Here's how the part is built. I have some questions about the finished solid (model axes, mm). A direction names the side the tool comes from. Round coordinates to 2 decimals unless told otherwise and drop trailing zeros. Write each loop counter-clockwise with the first axis right and the second up, starting at its lowest first coordinate (ties: lowest second). Pieces come first, ordered by that corner, then holes. Notation, with made-up numbers: (-31.75, -22) - (9.25, -22) arc R24 ccw to (9.25, 12) - close; hole circle Ø5 at (-10, -40). An arc over 180 degrees is marked (long way). Write item = value, one per line. Start each with the question number.
Item 1: Thinking about a two-plate mould opening in X: for faces 4 (the face through (10.57, 51.4, 1.52)), 5 (the face through (46, 39, 1)), 6 (the face through (28, 41.6, 1)), which applies, pulls with the +X half, pulls with the -X half, needs draft (parallel to the pull), parting line crosses it, or undercut?
Item 2: If we section it at D-D (x = 19): Please give me the cut outline in (y, z), and give its area (3 significant figures).
Item 3: If we section it at B-B (z = 10): Please give me the cut outline in (x, y).
Item 4: If we section it at A-A (y = 36.5): Please give me the cut outline in (x, z).
Item 5: Which directions (+Z, -Z, +X, -X, +Y, -Y) give clear straight access to the entire face, cutting with the end or side of a thin tool? Please do faces 1 (the face through (28, 31.6, 1)), 2 (the face through (54, 26, 6)), 3 (the face through (2, 26, 6)).
Item 6: If I drill on line 1 along Y through (x, z) = (2.1, 5); line 2 along X through (y, z) = (6.5, 7); line 3 along Z through (x, y) = (29, 45.5), over which ranges is the centre line in solid material (lowest first)? Write a range as [from, to].
Item 7: If we section it at C-C (z = 4.25): Please give me the cut outline in (x, y).
Item 8: For P1, Ø2, axis at y = 4, z = 5, coming from the +X side; P2, Ø6.5, axis at x = 5, z = 12, coming from the +Y side; P3, Ø0.9, axis at y = 35, z = 1, coming from the -X side; P4, Ø25, axis at x = 22.5, y = 14, coming from the +Z side, each with a flat end and sliding along its axis, tell me the tip position at first contact or that it passes through.
```python
from build123d import *

# Parameters (mm, degrees)
SKETCH_1_W          = 3
SKETCH_1_H          = 26
EXTRUDE_4_DEPTH     = 3
SKETCH_2_W          = 3
SKETCH_2_H          = 26
EXTRUDE_5_DEPTH     = 15
CUT_EXTRUDE_2_DEPTH = 56
FILLET_2_R          = 2


with BuildPart() as part:
    # 草图1 → 凸台-拉伸4 (new body)
    with BuildSketch(Plane.XY):
        with BuildLine():
            Line((10, 26), (3, 26))
            Line((3, 26), (3, 0))
            Line((3, 0), (28, 0))
            Line((28, 0), (28, 4.6))
            ThreePointArc((28, 4.6), (24.535898385, 5.110874707), (21.366750419, 6.6))
            Line((21.366750419, 6.6), (19.65, 6.6))
            ThreePointArc((19.65, 6.6), (16.833273811, 5.433273811), (18, 8.25))
            Line((18, 8.25), (18, 9.966750419))
            ThreePointArc((18, 9.966750419), (16, 16.6), (18, 23.233249581))
            Line((18, 23.233249581), (18, 24.95))
            ThreePointArc((18, 24.95), (16.35, 26.6), (18, 28.25))
            Line((18, 28.25), (18, 31.6))
            Line((18, 31.6), (18, 41.6))
            Line((18, 41.6), (18, 44.95))
            ThreePointArc((18, 44.95), (16.833273811, 47.766726189), (19.65, 46.6))
            Line((19.65, 46.6), (28, 46.6))
            Line((28, 46.6), (28, 52))
            Line((28, 52), (10, 52))
            Line((10, 52), (10, 26))
        make_face()
        with BuildLine():
            Line((28, 4.6), (28, 0))
            Line((28, 0), (53, 0))
            Line((53, 0), (53, 26))
            Line((53, 26), (46, 26))
            Line((46, 26), (46, 52))
            Line((46, 52), (28, 52))
            Line((28, 52), (28, 46.6))
            Line((28, 46.6), (36.35, 46.6))
            ThreePointArc((36.35, 46.6), (38, 48.25), (39.65, 46.6))
            ThreePointArc((39.65, 46.6), (39.166726189, 45.433273811), (38, 44.95))
            Line((38, 44.95), (38, 41.6))
            Line((38, 41.6), (38, 31.6))
            Line((38, 31.6), (38, 28.25))
            ThreePointArc((38, 28.25), (39.166726189, 27.766726189), (39.65, 26.6))
            ThreePointArc((39.65, 26.6), (39.166726189, 25.433273811), (38, 24.95))
            Line((38, 24.95), (38, 23.233249581))
            ThreePointArc((38, 23.233249581), (39.489125293, 20.064101615), (40, 16.6))
            ThreePointArc((40, 16.6), (39.489125293, 13.135898385), (38, 9.966750419))
            Line((38, 9.966750419), (38, 8.25))
            ThreePointArc((38, 8.25), (39.166726189, 7.766726189), (39.65, 6.6))
            ThreePointArc((39.65, 6.6), (38, 4.95), (36.35, 6.6))
            Line((36.35, 6.6), (34.633249581, 6.6))
            ThreePointArc((34.633249581, 6.6), (31.464101615, 5.110874707), (28, 4.6))
        make_face()
        with Locations((54.5, 13)):
            Rectangle(SKETCH_1_W, SKETCH_1_H)
        with Locations((1.5, 13)):
            Rectangle(SKETCH_1_W, SKETCH_1_H)
        with BuildLine():
            ThreePointArc((18, 23.233249581), (22.325451338, 27.173528147), (28, 28.6))
            Line((28, 28.6), (28, 31.6))
            Line((28, 31.6), (23, 31.6))
            Line((23, 31.6), (18, 31.6))
            Line((18, 31.6), (18, 28.25))
            ThreePointArc((18, 28.25), (19.166726189, 27.766726189), (19.65, 26.6))
            ThreePointArc((19.65, 26.6), (19.166726189, 25.433273811), (18, 24.95))
            Line((18, 24.95), (18, 23.233249581))
        make_face()
        with BuildLine():
            Line((28, 31.6), (28, 28.6))
            ThreePointArc((28, 28.6), (33.674548662, 27.173528147), (38, 23.233249581))
            Line((38, 23.233249581), (38, 24.95))
            ThreePointArc((38, 24.95), (36.35, 26.6), (38, 28.25))
            Line((38, 28.25), (38, 31.6))
            Line((38, 31.6), (28, 31.6))
        make_face()
        with BuildLine():
            Line((28, 41.6), (28, 46.6))
            Line((28, 46.6), (19.65, 46.6))
            ThreePointArc((19.65, 46.6), (19.166726189, 45.433273811), (18, 44.95))
            Line((18, 44.95), (18, 41.6))
            Line((18, 41.6), (28, 41.6))
        make_face()
        with BuildLine():
            Line((36.35, 46.6), (28, 46.6))
            Line((28, 46.6), (28, 41.6))
            Line((28, 41.6), (33, 41.6))
            Line((33, 41.6), (38, 41.6))
            Line((38, 41.6), (38, 44.95))
            ThreePointArc((38, 44.95), (36.833273811, 45.433273811), (36.35, 46.6))
        make_face()
    extrude(amount=EXTRUDE_4_DEPTH)

    # 草图2 → 凸台-拉伸5 (add)
    with BuildSketch(Plane.XY.offset(3)):
        with Locations((1.5, 13)):
            Rectangle(SKETCH_2_W, SKETCH_2_H)
        with Locations((54.5, 13)):
            Rectangle(SKETCH_2_W, SKETCH_2_H)
    extrude(amount=EXTRUDE_5_DEPTH)

    # 草图5 → 切除-拉伸2 (cut)
    with BuildSketch(Plane.ZY):
        with BuildLine():
            ThreePointArc((5, 10.35), (6.166726189, 10.833273811), (6.65, 12))
            Line((6.65, 12), (5, 12))
            Line((5, 12), (5, 10.35))
        make_face()
        with BuildLine():
            Line((5, 12), (6.65, 12))
            ThreePointArc((6.65, 12), (3.833273811, 13.166726189), (5, 10.35))
            Line((5, 10.35), (5, 12))
        make_face()
        with BuildLine():
            ThreePointArc((11.35, 12), (11.833273811, 10.833273811), (13, 10.35))
            Line((13, 10.35), (13, 12))
            Line((13, 12), (11.35, 12))
        make_face()
        with BuildLine():
            Line((13, 12), (13, 10.35))
            ThreePointArc((13, 10.35), (14.166726189, 10.833273811), (14.65, 12))
            ThreePointArc((14.65, 12), (13, 13.65), (11.35, 12))
            Line((11.35, 12), (13, 12))
        make_face()
        with BuildLine():
            ThreePointArc((6.65, 4), (6.166726189, 5.166726189), (5, 5.65))
            Line((5, 5.65), (5, 4))
            Line((5, 4), (6.65, 4))
        make_face()
        with BuildLine():
            Line((5, 4), (5, 5.65))
            ThreePointArc((5, 5.65), (3.833273811, 2.833273811), (6.65, 4))
            Line((6.65, 4), (5, 4))
        make_face()
        with BuildLine():
            ThreePointArc((14.65, 4), (14.166726189, 5.166726189), (13, 5.65))
            Line((13, 5.65), (13, 4))
            Line((13, 4), (11.35, 4))
            ThreePointArc((11.35, 4), (13, 2.35), (14.65, 4))
        make_face()
        with BuildLine():
            Line((13, 4), (13, 5.65))
            ThreePointArc((13, 5.65), (11.833273811, 5.166726189), (11.35, 4))
            Line((11.35, 4), (13, 4))
        make_face()
    extrude(amount=-CUT_EXTRUDE_2_DEPTH, mode=Mode.SUBTRACT)

    # 圆角2
    fillet_2_edges = [part.edges().sort_by_distance(p)[0] for p in [
        (46, 26, 1.5),
        (10, 26, 1.5),
        (10, 52, 1.5),
        (46, 52, 1.5),
        (1.5, 26, 18),
        (1.5, 0, 18),
        (54.5, 26, 18),
        (54.5, 0, 18),
    ]]
    fillet(fillet_2_edges, radius=FILLET_2_R)


solid = part.part
```
Reply:
q1.face_4 = pulls with the -X half
q1.face_5 = pulls with the +X half
q1.face_6 = undercut
q2.outline = (0, 0) - (5.29, 0) - (5.29, 3) - (0, 3) - close; (24.54, 0) - (25.29, 0) - (25.29, 3) - (24.54, 3) - close; (27.91, 0) - (31.6, 0) - (31.6, 3) - (27.91, 3) - close; (41.6, 0) - (45.29, 0) - (45.29, 3) - (41.6, 3) - close; (47.91, 0) - (52, 0) - (52, 3) - (47.91, 3) - close
q2.area = 52.5 mm2
q3.outline = (0, 0) - (3, 0) - (3, 26) - (0, 26) - close; (53, 0) - (56, 0) - (56, 26) - (53, 26) - close
q4.outline = (10, 0) - (18, 0) - (18, 3) - (10, 3) - close; (38, 0) - (46, 0) - (46, 3) - (38, 3) - close
q5.face_1 = +Z, -Z
q5.face_2 = +Z, -Z, +X, +Y
q5.face_3 = +Z, -Z, -X, +Y
q6.line_1 = [0, 2.35], [5.65, 10.35], [13.65, 26]
q6.line_2 = [0, 3], [53, 56]
q6.line_3 = [0, 3]
q7.outline = (0, 0) - (3, 0) - (3, 2.53) - (0, 2.53) - close; (0, 5.47) - (3, 5.47) - (3, 10.53) - (0, 10.53) - close; (0, 13.47) - (3, 13.47) - (3, 26) - (0, 26) - close; (53, 0) - (56, 0) - (56, 2.53) - (53, 2.53) - close; (53, 5.47) - (56, 5.47) - (56, 10.53) - (53, 10.53) - close; (53, 13.47) - (56, 13.47) - (56, 26) - (53, 26) - close
q8.P1 = through
q8.P2 = 26
q8.P3 = 10
q8.P4 = 3
